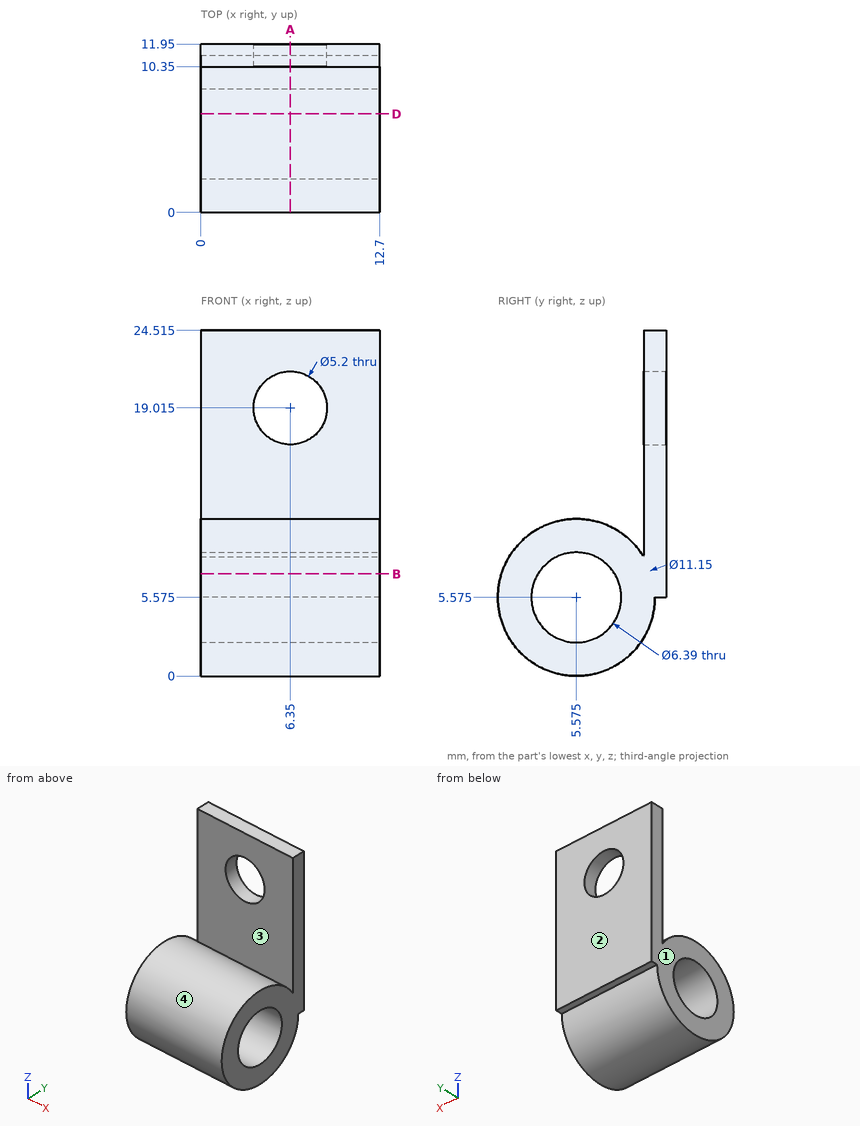
Answer from the drawing. Dimensions are ordinates in mm from the lowest x, y and z of the part. Round coordinates to 2 decimals unless told otherwise and drop trailing zeros. Write each loop counter-clockwise with the first axis right and the second up, starting at its lowest first coordinate (ties: lowest second). Pieces come first, ordered by that corner, then holes. Notation, with made-up numbers: M 6,54 L 24,54 A25 cw 24,75 Z; hole C 18.5,51 d1. An arc over 180 degrees is marked long. Write each question's results on one line, items separated by ' | '. Start each with the question number.
Item 1: Flat-ended cylindrical pins translate along their axes: pin 1 Ø7 at (x, z) = (6.35, 19.015) entering from -Y; pin 2 Ø6 at (x, y) = (2.5, 7) entering from +Z; pin 3 Ø4 at (x, y) = (7.5, 9) entering from -Z. Find the tip coordinate at first contact, or state that the pin passes through.
Item 2: A cutting plane is placed at B-B on z = 7.25. Write down the section's boundary in (x, y).
Item 3: For a pull along Y with two mould halves and no side action, classify the marked faces 1, 2, 3 and 4 as pulls with the +Y half, pulls with the -Y half, needs draft (parallel to the pull), parting line crosses it, or undercut.
Item 4: A cutting plane is placed at A-A on x = 6.35. State how many separate pieces and enclosed holes the cut face has, and give its area (3 significant figures).
Item 5: A cutting plane is placed at D-D on y = 7. Write down the section's boundary in (x, z), and give its area (3 significant figures).
Item 6: Straight lines are drawn through the part: L1, parallel to Y at x = 2.25, z = 5.5; L2, parallel to Z at x = 2, y = 5; L3, parallel to Z at x = 10, y = 11.5 (3 decimals). For each, find the intervals that lie inside material, in ascending order. Write a range as [from, to].
Check sheet entries:
1) pin 1: y = 10.35 | pin 2: z = 11.15 | pin 3: z = 0.19
2) outline: M 0,0.26 L 12.7,0.26 L 12.7,2.85 L 0,2.85 Z; M 0,8.3 L 12.7,8.3 L 12.7,11.95 L 0,11.95 Z
3) face 1: needs draft | face 2: pulls with the +Y half | face 3: undercut | face 4: undercut
4) separate pieces: 2 | enclosed holes: 1 | area: 86.0 mm²
5) outline: M 0,0.19 L 12.7,0.19 L 12.7,2.72 L 0,2.72 Z; M 0,8.43 L 12.7,8.43 L 12.7,10.96 L 0,10.96 Z | area: 64.3 mm²
6) L1: [0, 2.38], [8.77, 11.15] | L2: [0.03, 2.43], [8.72, 11.12] | L3: [5.575, 24.515]
